Part model, mm, in its own coordinate system. Face numbers are marked on the shaded views. A direction names the side the tool comes from. Give positions to 0.01 mm unless a question says otherwise; leave off trailing zeros. Order: outer loops, then holes, each group sorted by start corner. A loop starts at its lowest first (then second) coordinate and runs counter-clockwise, first axis right, second up. Notation, with made-up numbers: (14, 7) - (39, 7) arc R18 cw to (39, 17) - close; hole circle Ø8 at (-4.75, 78.5). An arc over 180 degrees is marked (long way). One line per item, written item: value.
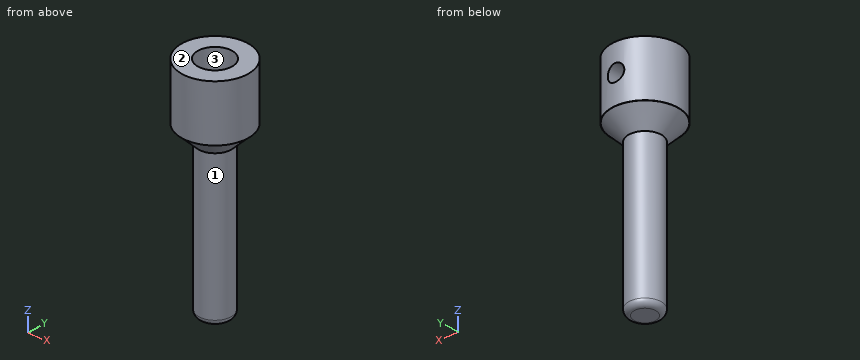
```python
from build123d import *

# Parameters (mm, degrees)
CYLINDER_R     = 1.49
CYLINDER_DEPTH = 20
SKETCH_R       = 6
PAD_DEPTH      = 10
SKETCH001_R    = 3.1
POCKET_DEPTH   = 7.5
SKETCH002_R    = 2.95
PAD001_DEPTH   = 30
FILLET_R       = 1
CHAMFER_SIZE   = 3


with BuildPart() as cilindro:
    # Cylinder → Cylinder (new body)
    with BuildSketch(Plane(origin=(0, 0, 5.2), x_dir=(1, 0, 0), z_dir=(0, 1, 0))):
        Circle(CYLINDER_R)
    extrude(amount=CYLINDER_DEPTH)


with BuildPart() as cut:
    # Sketch → Pad (new body)
    with BuildSketch(Plane.XY):
        Circle(SKETCH_R)
    extrude(amount=PAD_DEPTH)

    # Sketch001 (on Face3 of Pad) → Pocket (cut)
    with BuildSketch(Plane.XY.offset(10)):
        Circle(SKETCH001_R)
    extrude(amount=-POCKET_DEPTH, mode=Mode.SUBTRACT)

    # Sketch002 (on Face2 of Pocket) → Pad001 (join)
    with BuildSketch(Plane(origin=(0, 0, 0), x_dir=(1, 0, 0), z_dir=(0, 0, -1))):
        Circle(SKETCH002_R)
    extrude(amount=PAD001_DEPTH)

    # Fillet
    fillet_edges = [cut.edges().sort_by_distance(p)[0] for p in [
        (-2.95, 0, -30),
    ]]
    fillet(fillet_edges, radius=FILLET_R)

    # Chamfer
    chamfer_edges = [cut.edges().sort_by_distance(p)[0] for p in [
        (-2.95, 0, 0),
    ]]
    chamfer(chamfer_edges, length=CHAMFER_SIZE)

    # Cut: cut Cilindro
    add(cilindro.part, mode=Mode.SUBTRACT)


solid = cut.part
```
1) Which spindle directions (+Z, -Z, +X, -X, +Y, -Y) get a long thin tool onto all of the face, cutting with end or side? Do the marked faces 1, 2 and 3. Say none if no direction does.
Outcome:
face 1: -Z
face 2: +Z, +X, -X, +Y, -Y
face 3: +Z
2) Pin check, flat tips, straight feed: pin 1 (1.5 mm diameter, centred on y = 2.5, z = -14, fed in from -X); pin 2 (6 mm diameter, centred on x = 4, z = 4, fed in from -Y); pin 3 (3 mm diameter, centred on x = 1, y = -0.5, fed in from +Z); pin 4 (1.5 mm diameter, centred on x = 4, z = -26, fed in from -Y). Stop position of each tip, or through.
Outcome:
pin 1: stops at x = -2.37
pin 2: stops at y = -5.92
pin 3: stops at z = 2.5
pin 4: passes through
3) Cut at C-C, the plane z = -24. Give the cut face in (x, y), then the cut area to 3 significant figures.
Outcome:
outline: circle Ø5.9 at (0, 0)
area: 27.3 mm^2
4) Cut at D-D, the plane z = 5.2. Give the cut face in (x, y).
Outcome:
outline: (-1.49, 2.72) - (-1.49, 5.81) arc R6 ccw (long way) to (1.49, 5.81) - (1.49, 2.72) arc R3.1 cw (long way) to start
5) Cut at A-A, the plane x = 0. Give the cut face in (y, z).
Outcome:
outline: (-6, 0) - (-5.95, 0) - (-2.95, -3) - (-2.95, -29) arc R1 ccw to (-1.95, -30) - (1.95, -30) arc R1 ccw to (2.95, -29) - (2.95, -3) - (5.95, 0) - (6, 0) - (6, 3.71) - (3.1, 3.71) - (3.1, 2.5) - (-3.1, 2.5) - (-3.1, 10) - (-6, 10) - close; (3.1, 6.69) - (6, 6.69) - (6, 10) - (3.1, 10) - close
6) Drill centre lines: line 1 along Y through (x, z) = (0, 8.5); line 2 along X through (y, z) = (0, -7.5); line 3 along Z through (x, y) = (0, 3.75). Where is each one in solid material? Low to high. Write a range as from..to.
Outcome:
line 1: y = -6..-3.1, 3.1..6
line 2: x = -2.95..2.95
line 3: z = -2.2..3.71, 6.69..10
7) Cut at B-B, the plane y = 0. Give the cut face in (x, z).
Outcome:
outline: (-6, 0) - (-5.95, 0) - (-2.95, -3) - (-2.95, -29) arc R1 ccw to (-1.95, -30) - (1.95, -30) arc R1 ccw to (2.95, -29) - (2.95, -3) - (5.95, 0) - (6, 0) - (6, 10) - (3.1, 10) - (3.1, 2.5) - (-3.1, 2.5) - (-3.1, 10) - (-6, 10) - close
